The model under review builds one solid part; all positions refer to its coordinate system, in mm. Coordinates: 2 decimals unless noted, no trailing zeros. Write each loop counter-clockwise with the first axis right and the second up, starting at its lowest first coordinate (ties: lowest second). Pieces come first, ordered by that corner, then holes. Notation, with made-up numbers: M 0.5,32 L 34.5,32 A21 ccw 34.5,62 Z; hole C 16,56.25 d3. An arc over 180 degrees is marked long. Answer as a JSON object with one key per item and string values.
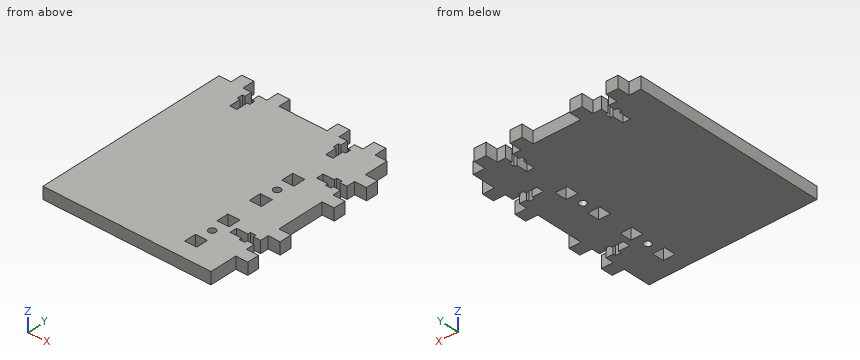
```python
from build123d import *

# Parameters (mm, degrees)
SKETCH1_R           = 1.5
SKETCH1_W           = 5
SKETCH1_H           = 5
BOSS_EXTRUDE1_DEPTH = 5


with BuildPart() as part:
    # Sketch1 → Boss-Extrude1 (new body)
    with BuildSketch(Plane.XY):
        Polygon((70, 81.5), (70, 71.5), (75, 71.5), (75, 66.5), (70, 66.5), (70, 63), (67, 63), (67, 64.1), (64.7, 64.1), (64.7, 63), (60, 63), (60, 60), (64.7, 60), (64.7, 58.9), (67, 58.9), (67, 60), (70, 60), (70, 56.5), (75, 56.5), (75, 51.5), (70, 51.5), (70, 31.5), (75, 31.5), (75, 26.5), (70, 26.5), (70, 23), (67, 23), (67, 24.1), (64.7, 24.1), (64.7, 23), (60, 23), (60, 20), (64.7, 20), (64.7, 18.9), (67, 18.9), (67, 20), (70, 20), (70, 16.5), (75, 16.5), (75, 11.5), (70, 11.5), (70, 0), (0, 0), (0, 81.5), (5, 81.5), (5, 86.5), (10, 86.5), (10, 81.5), (13.5, 81.5), (13.5, 78.5), (12.4, 78.5), (12.4, 76.2), (13.5, 76.2), (13.5, 71.5), (16.5, 71.5), (16.5, 76.2), (17.6, 76.2), (17.6, 78.5), (16.5, 78.5), (16.5, 81.5), (20, 81.5), (20, 86.5), (25, 86.5), (25, 81.5), (45, 81.5), (45, 86.5), (50, 86.5), (50, 81.5), (53.5, 81.5), (53.5, 78.5), (52.4, 78.5), (52.4, 76.2), (53.5, 76.2), (53.5, 71.5), (56.5, 71.5), (56.5, 76.2), (57.6, 76.2), (57.6, 78.5), (56.5, 78.5), (56.5, 81.5), (60, 81.5), (60, 86.5), (65, 86.5), (65, 81.5), align=None)
        with Locations((55.25, 47)):
            Circle(SKETCH1_R, mode=Mode.SUBTRACT)
        with Locations((55.25, 17)):
            Circle(SKETCH1_R, mode=Mode.SUBTRACT)
        with Locations((55.25, 39.5)):
            Rectangle(SKETCH1_W, SKETCH1_H, mode=Mode.SUBTRACT)
        with Locations((55.25, 54.5)):
            Rectangle(SKETCH1_W, SKETCH1_H, mode=Mode.SUBTRACT)
        with Locations((55.25, 9.5)):
            Rectangle(SKETCH1_W, SKETCH1_H, mode=Mode.SUBTRACT)
        with Locations((55.25, 24.5)):
            Rectangle(SKETCH1_W, SKETCH1_H, mode=Mode.SUBTRACT)
    extrude(amount=BOSS_EXTRUDE1_DEPTH)


solid = part.part
```
(1) Wall thickness on line 1 along X through (y, z) = (24, 4.5); line 2 along X through (y, z) = (73, 4.4); line 3 along X through (y, z) = (40.5, 4.8): over which ranges is each line inside the solid? List them lowest first. Write a range as from..to.
Results list:
{"line 1": "0..52.75, 57.75..64.7, 67..70", "line 2": "0..13.5, 16.5..53.5, 56.5..70", "line 3": "0..52.75, 57.75..70"}
(2) For pin 1 Ø1.5 at (x, z) = (56.5, 1.5) entering from +Y; pin 2 Ø2.5 at (y, z) = (85, 3.5) entering from +X; pin 3 Ø2.5 at (x, z) = (73.5, 1.5) entering from +Y, all flat-tipped, find the tip position at first contact; note any pin that passes through.
Results list:
{"pin 1": "y = 81.5", "pin 2": "x = 65", "pin 3": "y = 71.5"}
(3) Add section A-A on x = 55.25. Give the boundary of the cut face in (y, z), and give its area (4 significant figures).
Results list:
{"outline": "M 0,0 L 7,0 L 7,5 L 0,5 Z; M 12,0 L 15.5,0 L 15.5,5 L 12,5 Z; M 18.5,0 L 22,0 L 22,5 L 18.5,5 Z; M 27,0 L 37,0 L 37,5 L 27,5 Z; M 42,0 L 45.5,0 L 45.5,5 L 42,5 Z; M 48.5,0 L 52,0 L 52,5 L 48.5,5 Z; M 57,0 L 71.5,0 L 71.5,5 L 57,5 Z", "area": "227.5 mm²"}
(4) Add section B-B on y = 47. Give the boundary of the cut face in (x, z), and give its area (3 significant figures).
Results list:
{"outline": "M 0,0 L 53.75,0 L 53.75,5 L 0,5 Z; M 56.75,0 L 70,0 L 70,5 L 56.75,5 Z", "area": "335 mm²"}
(5) Add section D-D on z = 3.05. Count the separate pieces of the cut face and the enclosed holes in it, and give its area (3 significant figures).
Results list:
{"separate pieces": "1", "enclosed holes": "6", "area": "5,650 mm²"}
(6) Add section C-C on x = 68.5. Give the boundary of the cut face in (y, z).
Results list:
{"outline": "M 0,0 L 20,0 L 20,5 L 0,5 Z; M 23,0 L 60,0 L 60,5 L 23,5 Z; M 63,0 L 81.5,0 L 81.5,5 L 63,5 Z"}
